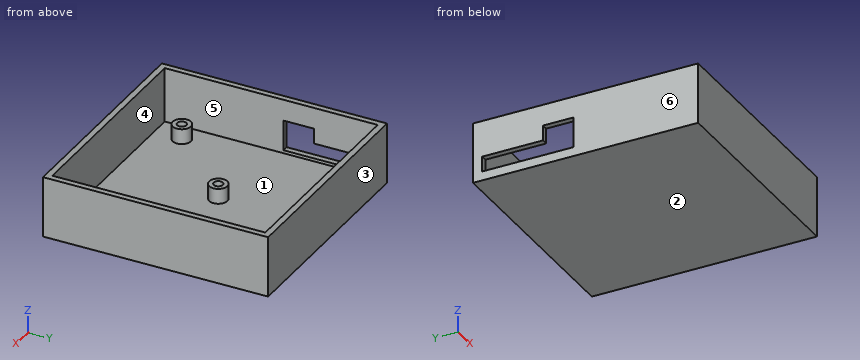
from build123d import *

# Parameters (mm, degrees)
SKETCH002_W     = 74
SKETCH002_H     = 74
PAD001_DEPTH    = 20
SKETCH003_W     = 70
SKETCH003_H     = 70
POCKET001_DEPTH = 18
SKETCH_R        = 3
PAD_DEPTH       = 5
SKETCH004_R     = 1.5
POCKET_DEPTH    = 5
POCKET002_DEPTH = 2


with BuildPart() as part:
    # Sketch002 → Pad001 (new body)
    with BuildSketch(Plane.XY):
        with Locations((37, 37)):
            Rectangle(SKETCH002_W, SKETCH002_H)
    extrude(amount=PAD001_DEPTH)

    # Sketch003 (on Face6 of Pad001) → Pocket001 (cut)
    with BuildSketch(Plane.XY.offset(20)):
        with Locations((37, 37)):
            Rectangle(SKETCH003_W, SKETCH003_H)
    extrude(amount=-POCKET001_DEPTH, mode=Mode.SUBTRACT)

    # Sketch (on Face11 of Pocket001) → Pad (join)
    with BuildSketch(Plane.XY.offset(2)):
        with Locations((8.52, 11.06)):
            Circle(SKETCH_R)
        with Locations((33.92, 36.46)):
            Circle(SKETCH_R)
        with Locations((64.4, 11.06)):
            Circle(SKETCH_R)
    extrude(amount=PAD_DEPTH)

    # Sketch004 (on Face17 of Pad) → Pocket (cut)
    with BuildSketch(Plane.XY.offset(7)):
        with Locations((8.52, 11.06)):
            Circle(SKETCH004_R)
        with Locations((64.4, 11.06)):
            Circle(SKETCH004_R)
        with Locations((33.92, 36.46)):
            Circle(SKETCH004_R)
    extrude(amount=-POCKET_DEPTH, mode=Mode.SUBTRACT)

    # Sketch005 (on Face2 of Pocket) → Pocket002 (cut)
    with BuildSketch(Plane(origin=(0, 0, 0), x_dir=(0, -1, 0), z_dir=(-1, 0, 0))):
        Polygon((-71, 8), (-71, 3), (-41, 3), (-41, 13), (-51, 13), (-51, 8), align=None)
    extrude(amount=-POCKET002_DEPTH, mode=Mode.SUBTRACT)


solid = part.part
Geometry: final body of the model. Coordinates: model frame, mm. Face numbers are marked on the shaded views. A direction names the side the tool comes from. Round coordinates to 2 decimals unless told otherwise and drop trailing zeros. Order: outer loops, then holes, each group sorted by start corner. A loop starts at its lowest first (then second) coordinate and runs counter-clockwise, first axis right, second up.
Q1. Section B-B, the plane x = 52. Output: boundary loops of the cut face in (y, z), and give its area (3 significant figures).
Result sheet:
outline: (0, 0) - (74, 0) - (74, 20) - (72, 20) - (72, 2) - (2, 2) - (2, 20) - (0, 20) - close
area: 220 mm2
Q2. Material intervals for probe 1 along Y at (x, z) = (61.5, 9.5); probe 2 along Y at (x, z) = (8, 2.75); probe 3 along Y at (x, z) = (8.52, 5.5), sorted ascending.
Result sheet:
probe 1: y = 0 to 2, 72 to 74
probe 2: y = 0 to 2, 8.11 to 9.65, 12.47 to 14.01, 72 to 74
probe 3: y = 0 to 2, 8.06 to 9.56, 12.56 to 14.06, 72 to 74
Q3. Mould query, pull axis Y, two halves, no side actions, for the marked faces 1, 2, 3 and 4. Classes: released by +Y, released by -Y, zero draft, split by the parting line, or undercut.
Result sheet:
face 1: undercut
face 2: zero draft
face 3: released by +Y
face 4: undercut
Q4. Section A-A, the plane y = 11.06. Output: boundary loops of the cut face in (x, z), and give its area (3 significant figures).
Result sheet:
outline: (0, 0) - (74, 0) - (74, 20) - (72, 20) - (72, 2) - (67.4, 2) - (67.4, 7) - (65.9, 7) - (65.9, 2) - (62.9, 2) - (62.9, 7) - (61.4, 7) - (61.4, 2) - (11.52, 2) - (11.52, 7) - (10.02, 7) - (10.02, 2) - (7.02, 2) - (7.02, 7) - (5.52, 7) - (5.52, 2) - (2, 2) - (2, 20) - (0, 20) - close
area: 250 mm2
Q5. Access query for the marked faces 5 and 6. Directions: +Z, -Z, +X, -X, +Y, -Y. A direction counts if a zero-diameter tool reaches every point of the face in a straight line with its end or side. Return the directions, or none.
Result sheet:
face 5: +Z
face 6: +Z, -Z, -X, +Y, -Y
Q6. Pin query (flat end, axial travel): pin 1 (5 mm diameter, centred on x = 7.5, y = 12, fed in from +Z); pin 2 (8 mm diameter, centred on x = 60, z = 5.5, fed in from -Y); pin 3 (1.5 mm diameter, centred on x = 9, y = 11.5, fed in from +Z). Return the tip coordinate at first contact, or that it passes through.
Result sheet:
pin 1: stops at z = 7
pin 2: stops at y = 0
pin 3: stops at z = 2
Q7. Section C-C, the plane y = 60. Output: boundary loops of the cut face in (x, z).
Result sheet:
outline: (0, 0) - (74, 0) - (74, 20) - (72, 20) - (72, 2) - (2, 2) - (2, 3) - (0, 3) - close; (0, 8) - (2, 8) - (2, 20) - (0, 20) - close
Q8. Section D-D, the plane z = 14.25. Output: boundary loops of the cut face in (x, y).
Result sheet:
outline: (0, 0) - (74, 0) - (74, 74) - (0, 74) - close; hole (2, 2) - (72, 2) - (72, 72) - (2, 72) - close
